Here's the drawing with two shaded views (mm, measured from the low corner). I have some questions. Give positions to 0.01 mm unless a question says otherwise; leave off trailing zeros. Write each loop counter-clockwise with the first axis right and the second up, starting at its lowest first coordinate (ties: lowest second). Pieces come first, ordered by that corner, then holes. Notation, with made-up numbers: M -32.75,1.25 L 20.25,1.25 A32 ccw 20.25,38.25 Z; hole C -11.5,17.5 d2. An arc over 180 degrees is marked long. Use one line per item in the form item = value.
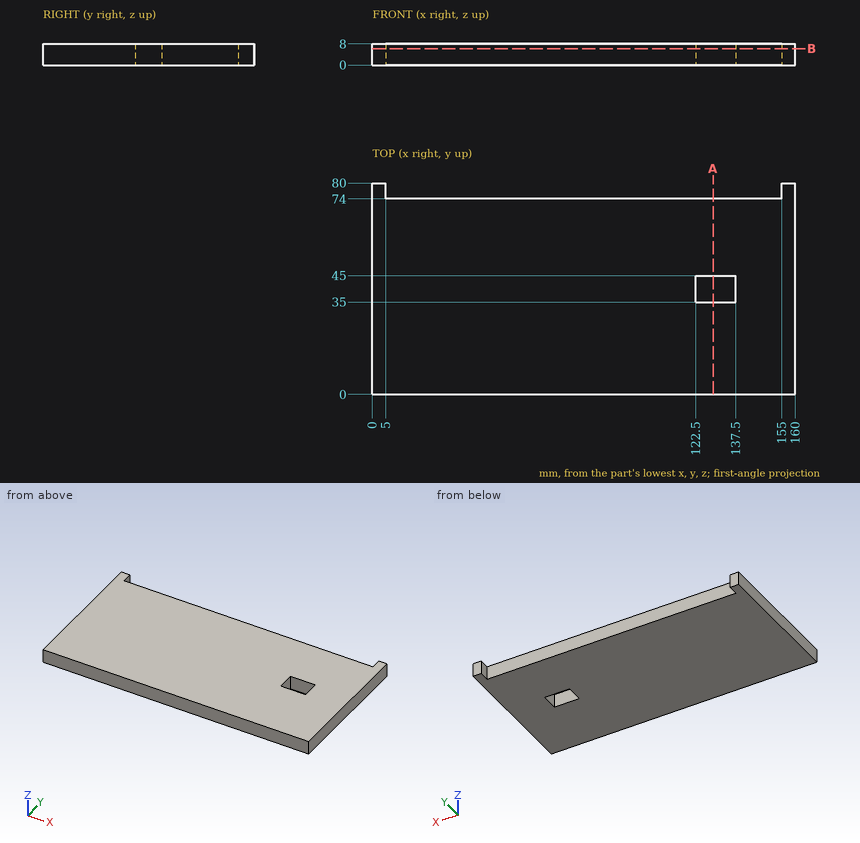
1) If I drill on L1, parallel to X at y = 40.5, z = 3.5; L2, parallel to X at y = 76, z = 6.5; L3, parallel to Y at x = 44, z = 3.5, over which ranges is the centre line in solid material (lowest first)?
Checked values:
L1 = 0 to 122.5, 137.5 to 160
L2 = 0 to 5, 155 to 160
L3 = 0 to 74
2) I want a section at A-A, the plane x = 129. Please give me the cut outline in (y, z), plus the area to 3 significant figures.
Checked values:
outline = M 0,0 L 35,0 L 35,8 L 0,8 Z; M 45,0 L 74,0 L 74,8 L 45,8 Z
area = 512 mm2
3) For pin 1 Ø2.5 at (x, z) = (103, 6) entering from +Y, with a flat end and sliding along its axis, tell me the tip position at first contact or that it passes through.
Checked values:
pin_1 = 74
4) I want a section at B-B, the plane z = 6.25. Please give me the cut outline in (x, y).
Checked values:
outline = M 0,0 L 160,0 L 160,80 L 155,80 L 155,74 L 5,74 L 5,80 L 0,80 Z; hole M 122.5,35 L 137.5,35 L 137.5,45 L 122.5,45 Z
